Verification items for the finished model (mm, model axes). A direction names the side the tool comes from. Give positions to 0.01 mm unless a question says otherwise; leave off trailing zeros. Loops run counter-clockwise (first coordinate to the right, second up) from the corner with the lowest first, then second, coordinate; pieces in that order, holes last. Notation, with made-up numbers: (-2, -5) - (42, -5) arc R8 cw to (42, 1) - close; hole circle Ø3 at (-33.75, 37.25). An arc over 180 degrees is marked (long way). One line per item, written item: value. Start each with the question number.
1. Sectioned sample at B-B (z = 18.75). Record the cut outline in (x, y), plus the area to 3 significant figures.
2. Gauge pin test, flat end, axial feed: pin 1 (4 mm diameter, centred on x = -14.5, y = 19.5, fed in from +Z). Record the tip position at first contact, or that the pin passes through.
3. Mould release check, pull along X, two halves, no side actions. Record for faces 1 (the flat face through (50.8, -1, 13)), 2 (the cylindrical face through (-13.592, -18.556, 7.727)), 3 (the flat face through (-12, 17, 0)): pulls with the +X half, pulls with the -X half, needs draft (parallel to the pull), parting line crosses it, or undercut.
4. Sectioned sample at A-A (z = 10.75). Record the cut outline in (x, y), plus the area to 3 significant figures.
5. Access from +Z, -Z, +X, -X, +Y, -Y to the whole of each face (thin tool, end or side, straight path). Record for faces 4 (the flat face through (-1, -38.1, 13)), 5 (the flat face through (19.576, -6.249, 7.513)), 6 (the cylindrical face through (-13.696, 19.031, 22.345)).
6. Scan lines: L1, parallel to X at y = -11.5, z = 23.75; L2, parallel to Y at x = -5, z = 8.5; L3, parallel to X at y = 17.5, z = 12.75. Record each from-to range of solid material in increasing order. Write a range as [from, to].
from build123d import *

# Parameters (mm, degrees)
F0_W     = 101.6
F0_H     = 76.2
F1_DEPTH = 25.4
F2_R     = 10.16


with BuildPart() as f1:
    # F0 (on Top) → F1 (new body)
    with BuildSketch(Plane.XY):
        Rectangle(F0_W, F0_H)
        Polygon((-24.156836, 7.849032), (0, 25.4), (24.156836, 7.849032), (14.929745, -20.549032), (-14.929745, -20.549032), align=None, mode=Mode.SUBTRACT)
    extrude(amount=F1_DEPTH)

    # F2
    f2_edges = [f1.edges().sort_by_distance(p)[0] for p in [
        (0, -20.549032, 25.4),
        (-19.54329, -6.35, 25.4),
        (-12.078418, 16.624516, 25.4),
        (12.078418, 16.624516, 25.4),
        (19.54329, -6.35, 25.4),
        (-14.929745, -20.549032, 12.7),
        (14.929745, -20.549032, 12.7),
        (24.156836, 7.849032, 12.7),
        (0, 25.4, 12.7),
        (-24.156836, 7.849032, 12.7),
    ]]
    fillet(f2_edges, radius=F2_R)


solid = f1.part
Results are:
1. outline: (-50.8, -38.1) - (50.8, -38.1) - (50.8, 38.1) - (-50.8, 38.1) - close; hole (-22.47, 0.64) - (-17.81, -13.72) arc R10.79 ccw to (-7.55, -21.17) - (7.55, -21.17) arc R10.79 ccw to (17.81, -13.72) - (22.47, 0.64) arc R10.79 ccw to (18.55, 12.69) - (6.34, 21.57) arc R10.79 ccw to (-6.34, 21.57) - (-18.55, 12.69) arc R10.79 ccw to start
1. area: 6,170 mm^2
2. pin 1: stops at z = 24.39
3. face 1: pulls with the +X half
3. face 2: undercut
3. face 3: needs draft
4. outline: (-50.8, -38.1) - (50.8, -38.1) - (50.8, 38.1) - (-50.8, 38.1) - close; hole (-21.88, 0.83) - (-17.21, -13.53) arc R10.16 ccw to (-7.55, -20.55) - (7.55, -20.55) arc R10.16 ccw to (17.21, -13.53) - (21.88, 0.83) arc R10.16 ccw to (18.18, 12.19) - (5.97, 21.06) arc R10.16 ccw to (-5.97, 21.06) - (-18.18, 12.19) arc R10.16 ccw to start
4. area: 6,260 mm^2
5. face 4: +Z, -Z, +X, -X, -Y
5. face 5: +Z, -Z
5. face 6: +Z
6. L1: x = [-50.8, -22.72], [22.72, 50.8]
6. L2: y = [-38.1, -20.55], [21.69, 38.1]
6. L3: x = [-50.8, -10.87], [10.87, 50.8]
